CAD build for the part. Positions are in the model's coordinates, mm. Face numbers are marked on the shaded views. A direction names the side the tool comes from. Round coordinates to 2 decimals unless told otherwise and drop trailing zeros. Write each loop counter-clockwise with the first axis right and the second up, starting at its lowest first coordinate (ties: lowest second). Pieces come first, ordered by that corner, then holes. Notation, with made-up numbers: (-6, -9) -> (47, -9) arc R24 ccw to (47, 24) -> close; hole circle Ø3 at (67.25, 45). An arc over 180 degrees is marked (long way). Answer in a Markdown table with one row per item. Add a question column.
```python
from build123d import *

# Parameters (mm, degrees)
BOSS_EXTRUDE1_DEPTH = 7.62
SKETCH2_R           = 1.778
CUT_EXTRUDE1_DEPTH  = 17.169449279
FILLET1_R           = 2.54
FILLET2_R           = 1.778
DRAFT1_ANGLE        = 5


with BuildPart() as part:
    # Sketch1 → Boss-Extrude1 (new body)
    with BuildSketch(Plane.XY):
        Polygon((-7.239, 0.9525), (-7.239, 3.1115), (7.239, 3.1115), (7.239, 0.9525), (14.097, 0.9525), (14.097, -1.0795), (5.207, -1.0795), (5.207, 1.0795), (-5.207, 1.0795), (-5.207, -1.0795), (-14.097, -1.0795), (-14.097, 0.9525), align=None)
    extrude(amount=BOSS_EXTRUDE1_DEPTH)

    # Sketch2 → Cut-Extrude1 (cut, through all)
    with BuildSketch(Plane(origin=(0, 0.9525, 0), x_dir=(1, 0, 0), z_dir=(0, 1, 0))):
        with Locations(Location((-10.668, -3.81, 0), (0, 0, 180))):
            Circle(SKETCH2_R)
        with Locations(Location((10.668, -3.81, 0), (0, 0, 180))):
            Circle(SKETCH2_R)
    extrude(amount=-CUT_EXTRUDE1_DEPTH, mode=Mode.SUBTRACT)

    # Fillet1
    fillet1_edges = [part.edges().sort_by_distance(p)[0] for p in [
        (-14.097, -0.0635, 0),
        (14.097, -0.0635, 0),
        (-14.097, -0.0635, 7.62),
        (14.097, -0.0635, 7.62),
    ]]
    fillet(fillet1_edges, radius=FILLET1_R)

    # Fillet2
    fillet2_edges = [part.edges().sort_by_distance(p)[0] for p in [
        (-7.239, 3.1115, 3.81),
        (7.239, 3.1115, 3.81),
    ]]
    fillet(fillet2_edges, radius=FILLET2_R)

    # Draft1
    draft1_faces = [part.faces().sort_by_distance(p)[0] for p in [
        (5.207, 0, 3.81),
        (-5.207, 0, 3.81),
    ]]
    draft(draft1_faces, Plane(origin=(-5.207, 1.0795, 7.62), x_dir=(0, 0, -1), z_dir=(0, -1, 0)), DRAFT1_ANGLE)


solid = part.part
```
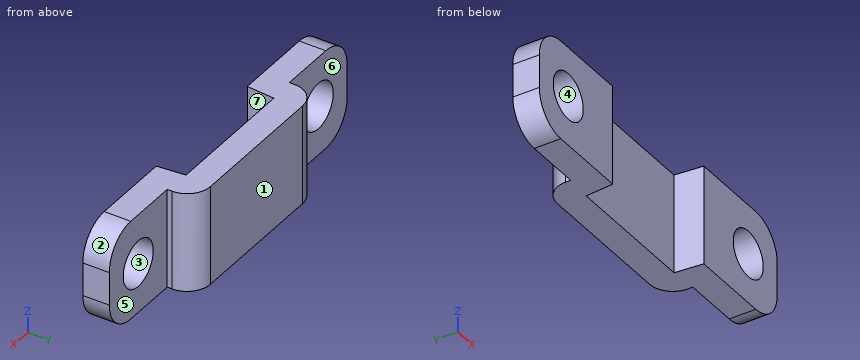
Item 1: Saw through at B-B on y = -0.2. Give the cut face in (x, z), then the cut area to 3 significant figures.
Item 2: Drill centre lines: probe 1 along X at (y, z) = (-0.7, 2.5); probe 2 along Y at (x, z) = (-2, 3.5); probe 3 along Y at (x, z) = (-9, 2.5). Where is each one in solid material? Low to high.
Item 3: Saw through at D-D on z = 7. Give the cut face in (x, y), then the cut area to 3 significant figures.
Item 4: Tool access for the marked faces 5, 6 and 7: list every direction of +Z, -Z, +X, -X, +Y, -Y with a clear straight run to the whole face (end or side of a thin tool).
Item 5: Saw through at C-C on x = 9.5. Give the cut face in (y, z), then the cut area to 3 significant figures.
Item 6: Pin check, flat tips, straight feed: pin 1 (1 mm diameter, centred on x = 2.5, z = 1.5, fed in from -Y); pin 2 (3.5 mm diameter, centred on x = 11, z = 5.5, fed in from +Y); pin 3 (2 mm diameter, centred on x = 10.668, z = 3.81, fed in from +Y). Stop position of each tip, or through.
Item 7: Two-plate mould, pull along Z, no slides. Class the marked faces 1, 2, 3 and 4: +Z half, -Z half, draft (parallel to the pull), parting line (faces both ways), or undercut.
Item 8: Saw through at A-A on z = 3.81. Give the cut face in (x, y).
Recorded:
| question | item | result |
|---|---|---|
| 1 | outline | (-14.1, 2.54) arc R2.54 ccw to (-11.56, 0) -> (-5.32, 0) -> (-5.32, 7.62) -> (-11.56, 7.62) arc R2.54 ccw to (-14.1, 5.08) -> close; (5.32, 0) -> (11.56, 0) arc R2.54 ccw to (14.1, 2.54) -> (14.1, 5.08) arc R2.54 ccw to (11.56, 7.62) -> (5.32, 7.62) -> close; hole circle Ø3.56 at (-10.67, 3.81); hole circle Ø3.56 at (10.67, 3.81) |
| 1 | area | 108 mm2 |
| 2 | probe 1 | -14.1 to -11.87, -9.47 to -5.36, 5.36 to 9.47, 11.87 to 14.1 |
| 2 | probe 2 | 1.08 to 3.11 |
| 2 | probe 3 | -1.08 to 0.95 |
| 3 | outline | (-13.22, -1.08) -> (-5.4, -1.08) -> (-5.21, 1.08) -> (5.21, 1.08) -> (5.4, -1.08) -> (13.22, -1.08) -> (13.22, 0.95) -> (7.24, 0.95) -> (7.24, 1.33) arc R1.78 ccw to (5.46, 3.11) -> (-5.46, 3.11) arc R1.78 ccw to (-7.24, 1.33) -> (-7.24, 0.95) -> (-13.22, 0.95) -> close |
| 3 | area | 60.7 mm2 |
| 4 | face 5 | +Z, -Z, +X, +Y |
| 4 | face 6 | +Z, -Z, -X, +Y |
| 4 | face 7 | +Z, -Z, -Y |
| 5 | outline | (-1.08, 0) -> (0.95, 0) -> (0.95, 2.47) -> (-1.08, 2.47) -> close; (-1.08, 5.15) -> (0.95, 5.15) -> (0.95, 7.62) -> (-1.08, 7.62) -> close |
| 5 | area | 10.0 mm2 |
| 6 | pin 1 | y = 1.08 |
| 6 | pin 2 | y = 0.95 |
| 6 | pin 3 | through |
| 7 | face 1 | draft |
| 7 | face 2 | +Z half |
| 7 | face 3 | undercut |
| 7 | face 4 | undercut |
| 8 | outline | (-14.1, -1.08) -> (-12.45, -1.08) -> (-12.45, 0.95) -> (-14.1, 0.95) -> close; (-8.89, -1.08) -> (-5.4, -1.08) -> (-5.21, 1.08) -> (5.21, 1.08) -> (5.4, -1.08) -> (8.89, -1.08) -> (8.89, 0.95) -> (7.24, 0.95) -> (7.24, 1.33) arc R1.78 ccw to (5.46, 3.11) -> (-5.46, 3.11) arc R1.78 ccw to (-7.24, 1.33) -> (-7.24, 0.95) -> (-8.89, 0.95) -> close; (12.45, -1.08) -> (14.1, -1.08) -> (14.1, 0.95) -> (12.45, 0.95) -> close |
